Read the model definition and answer for the solid it produces. Units are mm, in the model's axes. Face numbers are marked on the shaded views. Give positions to 0.01 mm unless a question says otherwise; leave off trailing zeros. Write each loop counter-clockwise with the first axis right and the second up, starting at its lowest first coordinate (ties: lowest second). Pieces come first, ordered by that corner, then holes. Notation, with made-up numbers: M -5.75,49 L 29.25,49 A28 ccw 29.25,71 Z; hole C 54,36 d4. An arc over 180 degrees is marked long. Use a Markdown table: item, result. Add a question column.
Item 1: A cutting plane is placed at A-A on x = 44.45. Determine the outline of the cut face in (y, z).
Item 2: Given P1, Ø1.9, axis at x = 44.5, z = 2.5, coming from the +Y side; P2, Ø4, axis at x = 56, y = 10.5, coming from the -Z side; P3, Ø3.5, axis at x = 51.5, z = 12.5, coming from the -Y side; P4, Ø8.5, axis at y = 26, z = 3.5, coming from the +X side, each flat-ended and moving along its own axis, determine where each tip first touches the part or whether it passes through.
Item 3: The mould has two halves that part along X. Classify the marked faces 1, 2 and 3: pulls with the +X half, pulls with the -X half, needs draft (parallel to the pull), parting line crosses it, or undercut.
Item 4: Consider probe 1 along X at (y, z) = (29, 2) (3 decimals); probe 2 along Z at (x, y) = (62.5, 6.5); probe 3 along X at (y, z) = (15, 7.5) (3 decimals). Determine where each line is inside the solid, lowest interval first. Write a range as [from, to].
Item 5: A cutting plane is placed at C-C on x = 24.5. Determine the outline of the cut face in (y, z).
Item 6: A cutting plane is placed at D-D on z = -20.5. Determine the outline of the cut face in (x, y), then the cut area to 3 significant figures.
from build123d import *

# Parameters (mm, degrees)
BOSS_EXTRUDE1_DEPTH = 76.2
BOSS_EXTRUDE2_DEPTH = 6.35
CUT_EXTRUDE1_DEPTH  = 6.35
SKETCH4_W           = 3.175
SKETCH4_H           = 25.4
BOSS_EXTRUDE3_DEPTH = 19.05


with BuildPart() as part:
    # Sketch1 → Boss-Extrude1 (new body)
    with BuildSketch(Plane(origin=(0, 0, 0), x_dir=(0, 0, -1), z_dir=(1, 0, 0))):
        Polygon((0, 0), (0, 63.5), (38.1, 63.5), (38.1, 61.9125), (1.5875, 61.9125), (1.5875, 0), align=None)
    extrude(amount=BOSS_EXTRUDE1_DEPTH)

    # Sketch2 → Boss-Extrude2 (add)
    with BuildSketch(Plane.XY):
        with BuildLine():
            Line((41.275, 12.7), (47.625, 12.7))
            ThreePointArc((47.625, 12.7), (49.87006403, 13.62993597), (50.8, 15.875))
            Line((50.8, 15.875), (50.8, 34.925))
            ThreePointArc((50.8, 34.925), (49.87006403, 37.17006403), (47.625, 38.1))
            Line((47.625, 38.1), (41.275, 38.1))
            ThreePointArc((41.275, 38.1), (39.02993597, 37.17006403), (38.1, 34.925))
            Line((38.1, 34.925), (38.1, 15.875))
            ThreePointArc((38.1, 15.875), (39.02993597, 13.62993597), (41.275, 12.7))
        make_face()
        with BuildLine():
            Line((41.275, 32.358201644), (41.275, 18.441798356))
            ThreePointArc((41.275, 18.441798356), (44.45, 15.266798356), (47.625, 18.441798356))
            Line((47.625, 18.441798356), (47.625, 32.358201644))
            ThreePointArc((47.625, 32.358201644), (44.45, 35.533201644), (41.275, 32.358201644))
        make_face(mode=Mode.SUBTRACT)
    extrude(amount=BOSS_EXTRUDE2_DEPTH)

    # Sketch3 → Cut-Extrude1 (cut)
    with BuildSketch(Plane.XY):
        with BuildLine():
            Line((47.625, 18.441798356), (47.625, 32.358201644))
            ThreePointArc((47.625, 32.358201644), (44.45, 35.533201644), (41.275, 32.358201644))
            Line((41.275, 32.358201644), (41.275, 18.441798356))
            ThreePointArc((41.275, 18.441798356), (44.45, 15.266798356), (47.625, 18.441798356))
        make_face()
    extrude(amount=-CUT_EXTRUDE1_DEPTH, mode=Mode.SUBTRACT)

    # Sketch4 → Boss-Extrude3 (add)
    with BuildSketch(Plane.XY):
        Polygon((50.8, 12.7), (50.8, 23.01875), (53.18125, 25.4), (53.975, 25.4), (53.975, 12.7), align=None)
        with Locations((36.5125, 25.4)):
            Rectangle(SKETCH4_W, SKETCH4_H)
    extrude(amount=BOSS_EXTRUDE3_DEPTH)


solid = part.part
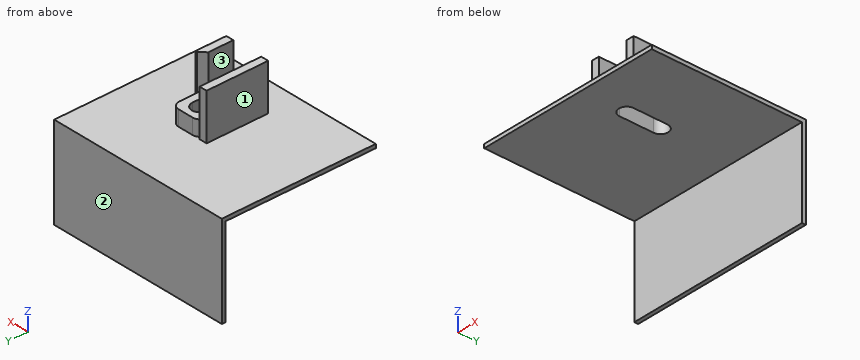
Filled in:
| question | item | result |
|---|---|---|
| 1 | outline | M 0,-1.59 L 15.27,-1.59 L 15.27,6.35 L 12.7,6.35 L 12.7,0 L 0,0 Z; M 35.53,-1.59 L 61.91,-1.59 L 61.91,-38.1 L 63.5,-38.1 L 63.5,0 L 38.1,0 L 38.1,6.35 L 35.53,6.35 Z |
| 2 | P1 | y = 38.1 |
| 2 | P2 | z = -1.59 |
| 2 | P3 | y = 12.7 |
| 2 | P4 | x = 76.2 |
| 3 | face 1 | pulls with the -X half |
| 3 | face 2 | needs draft |
| 3 | face 3 | undercut |
| 4 | probe 1 | [34.925, 41.275], [47.625, 50.8] |
| 4 | probe 2 | [-1.59, 0] |
| 4 | probe 3 | [34.925, 38.1], [50.8, 53.975] |
| 5 | outline | M 0,-1.59 L 61.91,-1.59 L 61.91,-38.1 L 63.5,-38.1 L 63.5,0 L 0,0 Z |
| 6 | outline | M 0,61.91 L 76.2,61.91 L 76.2,63.5 L 0,63.5 Z |
| 6 | area | 121 mm² |
